CAD build for the part. Positions are in the model's coordinates, mm. Coordinates: 2 decimals unless noted, no trailing zeros. Write each loop counter-clockwise with the first axis right and the second up, starting at its lowest first coordinate (ties: lowest second). Pieces come first, ordered by that corner, then holes. Notation, with made-up numbers: (-20, -33) -> (13, -33) arc R30 ccw to (13, 3) -> close; hole circle Ø5 at (9.5, 31.25). An arc over 180 degrees is marked (long way). Answer as CSV lines item,"result".
```python
from build123d import *

# Parameters (mm, degrees)
SKETCH1_R           = 4.88
BOSS_EXTRUDE1_DEPTH = 0.2
BOSS_EXTRUDE2_DEPTH = 0.001


with BuildPart() as part:
    # Sketch1 → Boss-Extrude1 (new body)
    with BuildSketch(Plane.XY):
        with Locations((-42.086326732, 0)):
            Circle(SKETCH1_R)
    extrude(amount=BOSS_EXTRUDE1_DEPTH)

    # Sketch2 → Boss-Extrude2 (add)
    with BuildSketch(Plane.XY.offset(0.2)):
        with BuildLine():
            Line((-41.120198615, 1.43163704), (-41.589950217, 1.001849379))
            add(Edge.make_bspline(
                [(-41.589950217, 1.001849379), (-41.610072362, 1.030233756), (-41.648704073, 1.084727801), (-41.711322047, 1.157696611), (-41.773657269, 1.219944437), (-41.836287237, 1.271211235), (-41.899767079, 1.311185521), (-41.963986602, 1.339487758), (-42.02858173, 1.357479758), (-42.071979684, 1.359720195), (-42.093355666, 1.360823738)],
                knots=[0, 0, 0, 0, 1.299362458, 2.494594718, 3.587462134, 4.587049575, 5.512617175, 6.380583204, 7.202344345, 8, 8, 8, 8], degree=3))
            add(Edge.make_bspline(
                [(-42.093355666, 1.360823738), (-42.113294569, 1.360124483), (-42.151791351, 1.358774403), (-42.20667137, 1.345354714), (-42.255394633, 1.322194302), (-42.297913587, 1.291910114), (-42.331594872, 1.255424689), (-42.358486766, 1.21716086), (-42.373629162, 1.174926245), (-42.3756222, 1.145917809), (-42.376608871, 1.131556912)],
                knots=[0, 0, 0, 0, 1.185010067, 2.2879431, 3.333075148, 4.379039566, 5.372662701, 6.27520591, 7.14612461, 8, 8, 8, 8], degree=3))
            add(Edge.make_bspline(
                [(-42.376608871, 1.131556912), (-42.375990574, 1.116988924), (-42.37474541, 1.087651022), (-42.362718816, 1.044652672), (-42.344591305, 1.002638279), (-42.327269728, 0.977062118), (-42.318415762, 0.963988803)],
                knots=[0, 0, 0, 0, 0.967525499, 1.948461899, 2.951351359, 4, 4, 4, 4], degree=3))
            add(Edge.make_bspline(
                [(-42.318415762, 0.963988803), (-42.31036655, 0.953827051), (-42.291838325, 0.930436041), (-42.256508796, 0.893388326), (-42.212142327, 0.848001634), (-42.157031604, 0.795836678), (-42.093464423, 0.735017403), (-42.018494364, 0.667934638), (-41.934279393, 0.592510908), (-41.874421342, 0.539988553), (-41.843055185, 0.512466367)],
                knots=[0, 0, 0, 0, 0.473873513, 1.090794244, 1.870441696, 2.795289791, 3.865433203, 5.087734844, 6.473946851, 8, 8, 8, 8], degree=3))
            add(Edge.make_bspline(
                [(-41.843055185, 0.512466367), (-41.813613535, 0.486986103), (-41.757739399, 0.438629857), (-41.678241599, 0.369995929), (-41.608376273, 0.308247658), (-41.547125643, 0.254311753), (-41.495418209, 0.207622303), (-41.453036591, 0.167956132), (-41.419463171, 0.136085468), (-41.400378648, 0.116835568), (-41.392233871, 0.108620213)],
                knots=[0, 0, 0, 0, 1.543621617, 2.929473131, 4.163658386, 5.240097082, 6.164993805, 6.925417477, 7.541396219, 8, 8, 8, 8], degree=3))
            add(Edge.make_bspline(
                [(-41.392233871, 0.108620213), (-41.361334287, 0.075180245), (-41.301934434, 0.010896882), (-41.224735565, -0.088722113), (-41.161198399, -0.185970564), (-41.112044842, -0.28267836), (-41.074922099, -0.380240801), (-41.048750074, -0.481050601), (-41.033075474, -0.58616116), (-41.031335227, -0.657886284), (-41.030455025, -0.694164242)],
                knots=[0, 0, 0, 0, 1.206664779, 2.319633467, 3.337109185, 4.282041471, 5.190008762, 6.099243693, 7.03861361, 8, 8, 8, 8], degree=3))
            add(Edge.make_bspline(
                [(-41.030455025, -0.694164242), (-41.03108153, -0.729512664), (-41.032310757, -0.798867582), (-41.047366424, -0.900358175), (-41.068834923, -0.997489076), (-41.102028988, -1.089203366), (-41.142485717, -1.177006505), (-41.193204071, -1.2595308), (-41.252765823, -1.337611431), (-41.321032735, -1.409852611), (-41.396544047, -1.475406475), (-41.477537106, -1.533764073), (-41.564803902, -1.581945703), (-41.657598842, -1.621619839), (-41.755872254, -1.652177389), (-41.859507066, -1.674762266), (-41.968661794, -1.688317354), (-42.043303369, -1.689734377), (-42.081436596, -1.690458313)],
                knots=[0, 0, 0, 0, 1.043214005, 2.046824704, 3.02475056, 3.976699089, 4.921714032, 5.875962561, 6.831408892, 7.817874052, 8.806269674, 9.781291748, 10.760897367, 11.74438705, 12.757449933, 13.795994037, 14.874007457, 16, 16, 16, 16], degree=3))
            add(Edge.make_bspline(
                [(-42.081436596, -1.690458313), (-42.111370853, -1.689927259), (-42.170657851, -1.688875468), (-42.258037922, -1.680288472), (-42.342413259, -1.666429973), (-42.42368882, -1.646566604), (-42.502230766, -1.621397021), (-42.578042322, -1.59065334), (-42.650600136, -1.553859045), (-42.720453215, -1.511770773), (-42.787261986, -1.462900746), (-42.851871221, -1.408248094), (-42.913639159, -1.346972236), (-42.972862459, -1.279218087), (-43.029162194, -1.204793783), (-43.084381256, -1.124735821), (-43.136065543, -1.037558433), (-43.167993227, -0.97640279), (-43.184301179, -0.945165845)],
                knots=[0, 0, 0, 0, 1.016823716, 2.013894106, 2.979844003, 3.91962641, 4.853723003, 5.779685073, 6.695824784, 7.614987388, 8.547259901, 9.504950863, 10.487499108, 11.500346958, 12.559593716, 13.656357062, 14.802919212, 16, 16, 16, 16], degree=3))
            Line((-43.184301179, -0.945165845), (-42.631817205, -0.613535236))
            add(Edge.make_bspline(
                [(-42.631817205, -0.613535236), (-42.611418394, -0.64899325), (-42.572312131, -0.716969293), (-42.506042911, -0.808303722), (-42.438153479, -0.886516541), (-42.367074292, -0.950225336), (-42.293669645, -1.000281972), (-42.217584977, -1.036055918), (-42.138766834, -1.058199949), (-42.085079495, -1.060904247), (-42.058299576, -1.062253185)],
                knots=[0, 0, 0, 0, 1.283663364, 2.460892379, 3.537111102, 4.529833553, 5.449777664, 6.316464042, 7.160231139, 8, 8, 8, 8], degree=3))
            add(Edge.make_bspline(
                [(-42.058299576, -1.062253185), (-42.031060565, -1.061151569), (-41.978212917, -1.059014274), (-41.902779662, -1.039272727), (-41.833619597, -1.00827705), (-41.773838148, -0.964050493), (-41.723218986, -0.913006324), (-41.685859139, -0.856217352), (-41.662389431, -0.794773055), (-41.659908114, -0.752089805), (-41.658660153, -0.730622576)],
                knots=[0, 0, 0, 0, 1.13588714, 2.203786484, 3.234766741, 4.283437687, 5.291419208, 6.222934724, 7.106237994, 8, 8, 8, 8], degree=3))
            add(Edge.make_bspline(
                [(-41.658660153, -0.730622576), (-41.659812594, -0.710650812), (-41.662153666, -0.670080087), (-41.679397282, -0.609757943), (-41.706354313, -0.549463231), (-41.738246381, -0.500007878), (-41.770700555, -0.458600251), (-41.801734064, -0.422722416), (-41.83952467, -0.383083689), (-41.883976551, -0.339634207), (-41.934502382, -0.291991475), (-41.991144725, -0.240160157), (-42.054552194, -0.184596825), (-42.099368718, -0.146747633), (-42.122802781, -0.12695671)],
                knots=[0, 0, 0, 0, 0.916159276, 1.861089862, 2.860218735, 3.940849679, 4.552606315, 5.27541173, 6.11797699, 7.06649574, 8.129236253, 9.306560635, 10.591630461, 12, 12, 12, 12], degree=3))
            add(Edge.make_bspline(
                [(-42.122802781, -0.12695671), (-42.167351868, -0.089263911), (-42.252855049, -0.016920021), (-42.373681891, 0.089929627), (-42.482557695, 0.189790414), (-42.578542091, 0.283896837), (-42.662858071, 0.370510968), (-42.734934608, 0.450336322), (-42.79397991, 0.52398864), (-42.856112359, 0.611224883), (-42.915150608, 0.717528239), (-42.966176408, 0.845423499), (-42.999279794, 0.973302532), (-43.002988568, 1.059153471), (-43.004813999, 1.101408674)],
                knots=[0, 0, 0, 0, 1.345494975, 2.582412109, 3.71882943, 4.751509156, 5.681369928, 6.505683931, 7.230279997, 7.856715994, 8.973648664, 10.023341002, 11.027102913, 12, 12, 12, 12], degree=3))
            add(Edge.make_bspline(
                [(-43.004813999, 1.101408674), (-43.004054805, 1.131373797), (-43.00255911, 1.190408307), (-42.989217283, 1.277209952), (-42.969277414, 1.360966246), (-42.940318999, 1.441371608), (-42.902734473, 1.518325328), (-42.857089527, 1.592204125), (-42.80267538, 1.662328036), (-42.74135431, 1.728650574), (-42.67379419, 1.789261826), (-42.601597617, 1.842757329), (-42.525173229, 1.887940409), (-42.444988552, 1.925423055), (-42.360546715, 1.954113639), (-42.272469796, 1.974450955), (-42.180631467, 1.986546942), (-42.118165017, 1.988191251), (-42.086344448, 1.989028867)],
                knots=[0, 0, 0, 0, 1.010766082, 1.991317756, 2.957454644, 3.913069143, 4.869106762, 5.843196583, 6.838735724, 7.860187025, 8.887984031, 9.89767229, 10.887916223, 11.879572884, 12.879850636, 13.892031539, 14.926195476, 16, 16, 16, 16], degree=3))
            add(Edge.make_bspline(
                [(-42.086344448, 1.989028867), (-42.045106566, 1.987520297), (-41.962956318, 1.984515066), (-41.841494807, 1.961015141), (-41.722856281, 1.924059033), (-41.627255134, 1.879475555), (-41.551187086, 1.836287519), (-41.492888033, 1.796525416), (-41.433565608, 1.750975789), (-41.372741413, 1.699495101), (-41.311545656, 1.641113386), (-41.248238248, 1.577220469), (-41.183681831, 1.507264164), (-41.141730396, 1.457287704), (-41.120198615, 1.43163704)],
                knots=[0, 0, 0, 0, 1.282922637, 2.555718331, 3.837320111, 5.142675274, 5.830281639, 6.55870424, 7.337177975, 8.157850921, 9.037902056, 9.96903443, 10.957596896, 12, 12, 12, 12], degree=3))
        make_face()
    extrude(amount=BOSS_EXTRUDE2_DEPTH)


solid = part.part
```
Item 1: Saw through at B-B on x = -38.5. Give the cut face in (y, z), and give its area (3 significant figures).
Answer below:
outline,"(-3.31, 0) -> (3.31, 0) -> (3.31, 0.2) -> (-3.31, 0.2) -> close"
area,"1.32 mm2"
Item 2: Wall check: line 1 (Z direction, x = -40.5, y = -2); line 2 (Y direction, x = -42.5, z = 0.1); line 3 (X direction, y = -0.5, z = 0.15). Give the ranges that are in metal, low to high. Write a range as from..to.
Answer below:
line 1,"z = 0..0.2"
line 2,"y = -4.86..4.86"
line 3,"x = -46.94..-37.23"
Item 3: Saw through at A-A on z = 0.05. Give the cut face in (x, y).
Answer below:
outline,"circle Ø9.76 at (-42.09, 0)"
Item 4: Saw through at C-C on y = 3.25. Give the cut face in (x, z), and give its area (3 significant figures).
Answer below:
outline,"(-45.73, 0) -> (-38.45, 0) -> (-38.45, 0.2) -> (-45.73, 0.2) -> close"
area,"1.46 mm2"
Item 5: Flat gauge pin, fed straight in: pin 1 (1 mm diameter, centred on x = -44, y = 0, fed in from -Z). Where does the tip first touch, or does it go through?
Answer below:
pin 1,"stops at z = 0"
